```python
from build123d import *

# Parameters (mm, degrees)
SKETCH1_R           = 4
SKETCH1_R_2         = 1.6
BOSS_EXTRUDE1_DEPTH = 8
FILLET1_R           = 1


with BuildPart() as part:
    # Sketch1 → Boss-Extrude1 (new body)
    with BuildSketch(Plane(origin=(0, 0, 0), x_dir=(1, 0, 0), z_dir=(0, 1, 0))):
        Circle(SKETCH1_R)
        Circle(SKETCH1_R_2, mode=Mode.SUBTRACT)
    extrude(amount=BOSS_EXTRUDE1_DEPTH)

    # Fillet1
    fillet1_edges = [part.edges().sort_by_distance(p)[0] for p in [
        (-4, 0, 0),
        (-4, 8, 0),
        (-1.6, 8, 0),
    ]]
    fillet(fillet1_edges, radius=FILLET1_R)


solid = part.part
```
The model under review builds one solid part; all positions refer to its coordinate system, in mm. Give positions to 0.01 mm unless a question says otherwise; leave off trailing zeros. Order: outer loops, then holes, each group sorted by start corner. A loop starts at its lowest first (then second) coordinate and runs counter-clockwise, first axis right, second up. Notation, with made-up numbers: (71, 26) - (118, 26) arc R29 ccw to (118, 48) - close; hole circle Ø11 at (-10, -28). An arc over 180 degrees is marked (long way). Use CSV: the item, a comma, the result in double quotes. Start each with the question number.
Q1. We need section C-C, the plane y = 1.75. Write out the cut boundary in (x, z).
Q2. To check wall thickness, follow line 1 along Z through (x, y) = (0, 4); line 2 along Z through (x, y) = (1.25, 1). State the ranges of each line that lie inside material, in increasing order. Write a range as [from, to].
Q3. The part is to be moulded in two halves that separate along Z. For faces 1 (the flat face through (1.3, 0, 1.3)), 2 (the cylindrical face through (-0.867, 3.958, 3.905)), 3 (the cylindrical face through (-1.27, 3.45, 0.97)), say which applies: +Z half, -Z half, draft (parallel to the pull), parting line (faces both ways), or undercut.
Q4. Clearance check with a flat-ended pin moving along its axis: pin 1 Ø1 at (y, z) = (6.5, 2.5) entering from -X. State where the tip first meets the part, or that it passes through.
Q5. We need section B-B, the plane z = 0. Write out the cut boundary in (x, y), and give its area (3 significant figures).
Q6. We need section A-A, the plane x = 0. Write out the cut boundary in (y, z), and give its area (3 significant figures).
Outcome:
1,outline,"circle Ø8 at (0, 0); hole circle Ø3.2 at (0, 0)"
2,line 1,"z = [-4, -1.6], [1.6, 4]"
2,line 2,"z = [-3.8, -1], [1, 3.8]"
3,face 1,"draft"
3,face 2,"parting line"
3,face 3,"undercut"
4,pin 1,"stops at x = -3.46"
5,outline,"(-4, 1) arc R1 ccw to (-3, 0) - (-1.6, 0) - (-1.6, 7) arc R1 ccw to (-2.6, 8) - (-3, 8) arc R1 ccw to (-4, 7) - close; (1.6, 0) - (3, 0) arc R1 ccw to (4, 1) - (4, 7) arc R1 ccw to (3, 8) - (2.6, 8) arc R1 ccw to (1.6, 7) - close"
5,area,"37.1 mm^2"
6,outline,"(0, -3) arc R1 ccw to (1, -4) - (7, -4) arc R1 ccw to (8, -3) - (8, -2.6) arc R1 ccw to (7, -1.6) - (0, -1.6) - close; (0, 1.6) - (7, 1.6) arc R1 ccw to (8, 2.6) - (8, 3) arc R1 ccw to (7, 4) - (1, 4) arc R1 ccw to (0, 3) - close"
6,area,"37.1 mm^2"
